Verification items for the finished model (mm, model axes). A direction names the side the tool comes from. Coordinates: 2 decimals unless noted, no trailing zeros. Order: outer loops, then holes, each group sorted by start corner. A loop starts at its lowest first (then second) coordinate and runs counter-clockwise, first axis right, second up. Notation, with made-up numbers: M -22.5,-36.5 L -1.5,-36.5 A15 cw -1.5,-24.5 Z; hole C 42.25,45.25 d6. An arc over 180 degrees is marked long. Return JSON: item names as keys, results as strings.
```python
from build123d import *

# Parameters (mm, degrees)
SKETCH1_W           = 25
SKETCH1_H           = 25
BOSS_EXTRUDE1_DEPTH = 25
SKETCH2_W           = 12
SKETCH2_H           = 10
BOSS_EXTRUDE2_DEPTH = 10
BOSS_EXTRUDE4_DEPTH = 2
LPATTERN1_COUNT     = 15
LPATTERN1_PITCH     = 0.96
CUT_EXTRUDE1_REACH  = 43.908
SKETCH4_W           = 0.720746126
SKETCH4_H           = 14.030445764
SKETCH5_W           = 10.5
SKETCH5_H           = 0.72
CUT_EXTRUDE2_DEPTH  = 14.3
CUT_EXTRUDE3_DEPTH  = 0.72
BOSS_EXTRUDE5_REACH = 40.386
SKETCH8_W           = 0.72
SKETCH8_H           = 0.3
SKETCH10_W          = 0.720746126
SKETCH10_H          = 0.030490047
BOSS_EXTRUDE6_DEPTH = 4


with BuildPart() as part:
    # Sketch1 → Boss-Extrude1 (new body)
    with BuildSketch(Plane(origin=(0, 0, 0), x_dir=(1, 0, 0), z_dir=(0, 1, 0))):
        Rectangle(SKETCH1_W, SKETCH1_H)
    extrude(amount=BOSS_EXTRUDE1_DEPTH)

    # Sketch2 → Boss-Extrude2 (add)
    with BuildSketch(Plane.XY.offset(12.5)):
        with Locations((0, 6)):
            Rectangle(SKETCH2_W, SKETCH2_H)
    extrude(amount=BOSS_EXTRUDE2_DEPTH)

    # Sketch3 → Boss-Extrude4 (add, symmetric)
    with BuildSketch(Plane(origin=(0, 0, 0), x_dir=(0, 0, -1), z_dir=(1, 0, 0))):
        Polygon((-12.5, 25), (-12.5, 24.2574888), (-13.297852918, 24.6287444), align=None)
    boss_extrude4 = extrude(amount=BOSS_EXTRUDE4_DEPTH, both=True)

    # LPattern1: Boss-Extrude4 ×15
    with Locations(*[(0, -i * LPATTERN1_PITCH, 0) for i in range(1, LPATTERN1_COUNT)]):
        add(boss_extrude4)

    # Cut-Extrude1: up to this face of the body (flat: up to its plane)
    cut_extrude1_end = Plane(part.part.faces().sort_by_distance((2, 24.6287444, 12.765950973))[0])
    # Sketch4 → Cut-Extrude1 (cut, up to the picked face)
    with BuildSketch(Plane(origin=(12.5, 0, 0), x_dir=(0, 0, -1), z_dir=(1, 0, 0)), mode=Mode.PRIVATE) as cut_extrude1_sk1:
        with Locations((-12.139626937, 17.984777118)):
            Rectangle(SKETCH4_W, SKETCH4_H)
    cut_extrude1_tool1 = split(extrude(cut_extrude1_sk1.sketch, amount=-CUT_EXTRUDE1_REACH, mode=Mode.PRIVATE), bisect_by=cut_extrude1_end, keep=Keep.BOTH, mode=Mode.PRIVATE)
    add(cut_extrude1_tool1.solids().sort_by(Axis((12.5, 17.984777, 12.139627), (-1, 0, 0)))[0], mode=Mode.SUBTRACT)

    # Sketch5 → Cut-Extrude2 (cut)
    with BuildSketch(Plane(origin=(0, 25, 0), x_dir=(1, 0, 0), z_dir=(0, 1, 0))):
        with Locations((-7.25, -12.14)):
            Rectangle(SKETCH5_W, SKETCH5_H)
    extrude(amount=-CUT_EXTRUDE2_DEPTH, mode=Mode.SUBTRACT)

    # Sketch7 → Cut-Extrude3 (cut)
    with BuildSketch(Plane.XY.offset(12.5)):
        Polygon((-6, 10.7), (-12.5, 10.7), (-12.5, 0), (12.5, 0), (12.5, 10.969554236), (6, 10.969554236), (6, 1), (-6, 1), align=None)
    extrude(amount=-CUT_EXTRUDE3_DEPTH, mode=Mode.SUBTRACT)

    # Sketch8 → Boss-Extrude5 (add, up to next)
    with BuildSketch(Plane.ZY.offset(6), mode=Mode.PRIVATE) as boss_extrude5_sk1:
        with Locations((12.14, 10.85)):
            Rectangle(SKETCH8_W, SKETCH8_H)
    boss_extrude5_tool1 = extrude(boss_extrude5_sk1.sketch, amount=-BOSS_EXTRUDE5_REACH, mode=Mode.PRIVATE) - part.part
    add(boss_extrude5_tool1.solids().sort_by_distance((-6, 10.85, 12.14))[0])

    # Sketch10 → Boss-Extrude6 (add)
    with BuildSketch(Plane(origin=(2, 0, 0), x_dir=(0, 0, -1), z_dir=(1, 0, 0))):
        with Locations((-12.139626937, 10.98479926)):
            Rectangle(SKETCH10_W, SKETCH10_H)
    extrude(amount=BOSS_EXTRUDE6_DEPTH)


solid = part.part
```
Q1. Cross-section at A-A, the plane x = -5. Record the boundary of the cut face in (y, z).
Values:
{"outline": "M 0,-12.5 L 25,-12.5 L 25,11.78 L 11,11.78 L 11,22.5 L 1,22.5 L 1,11.78 L 0,11.78 Z"}
Q2. Go/stop test with flat-tipped pins: pin 1 (12 mm diameter, centred on x = -1.5, z = 18.5, fed in from -Y); pin 2 (2 mm diameter, centred on x = 9.5, y = 14.5, fed in from +Z); pin 3 (8 mm diameter, centred on y = 4.5, z = 18, fed in from -X); pin 4 (8 mm diameter, centred on y = 16.5, z = 12.5, fed in from +X). Record where each tip stops, or that it passes through.
Values:
{"pin 1": "y = 1", "pin 2": "z = 11.78", "pin 3": "x = -6", "pin 4": "x = 12.5"}
Q3. Draft check along Y on faces 4 (the face through (0, 6, 22.5)), 5 (the face through (0, 25, 0)), 6 (the face through (0, 1, 17)). Enter one of: pulls with the +Y half, pulls with the -Y half, needs draft (parallel to the pull), parting line crosses it, or undercut.
Values:
{"face 4": "needs draft", "face 5": "pulls with the +Y half", "face 6": "pulls with the -Y half"}
Q4. Cross-section at C-C, the plane z = 15.5. Record the boundary of the cut face in (x, y), and give its area (3 significant figures).
Values:
{"outline": "M -6,1 L 6,1 L 6,11 L -6,11 Z", "area": "120 mm^2"}
Q5. Material ranges on line 1 along Z through (x, y) = (-6.5, 11.25); line 2 along X through (y, z) = (5, 16); line 3 along Y through (x, z) = (1.25, 17.5), recorded low to high.
Values:
{"line 1": "-12.5 to 11.78", "line 2": "-6 to 6", "line 3": "1 to 11"}
Q6. Cross-section at B-B, the plane y = 4.5. Record the boundary of the cut face in (x, z), and give its area (3 significant figures).
Values:
{"outline": "M -12.5,-12.5 L 12.5,-12.5 L 12.5,11.78 L 6,11.78 L 6,22.5 L -6,22.5 L -6,11.78 L -12.5,11.78 Z", "area": "736 mm^2"}
Q7. Tool access check on faces 1 (the face through (-6, 6, 17)), 2 (the face through (6, 6, 17)), 3 (the face through (2, 18, 12)). Record the directions out of +Z, -Z, +X, -X, +Y, -Y that give a thin tool (end or side, any length) a straight path to the whole face; none if there is none.
Values:
{"face 1": "+Z, -X, +Y, -Y", "face 2": "+Z, +X, +Y, -Y", "face 3": "+Z, +X, +Y"}
